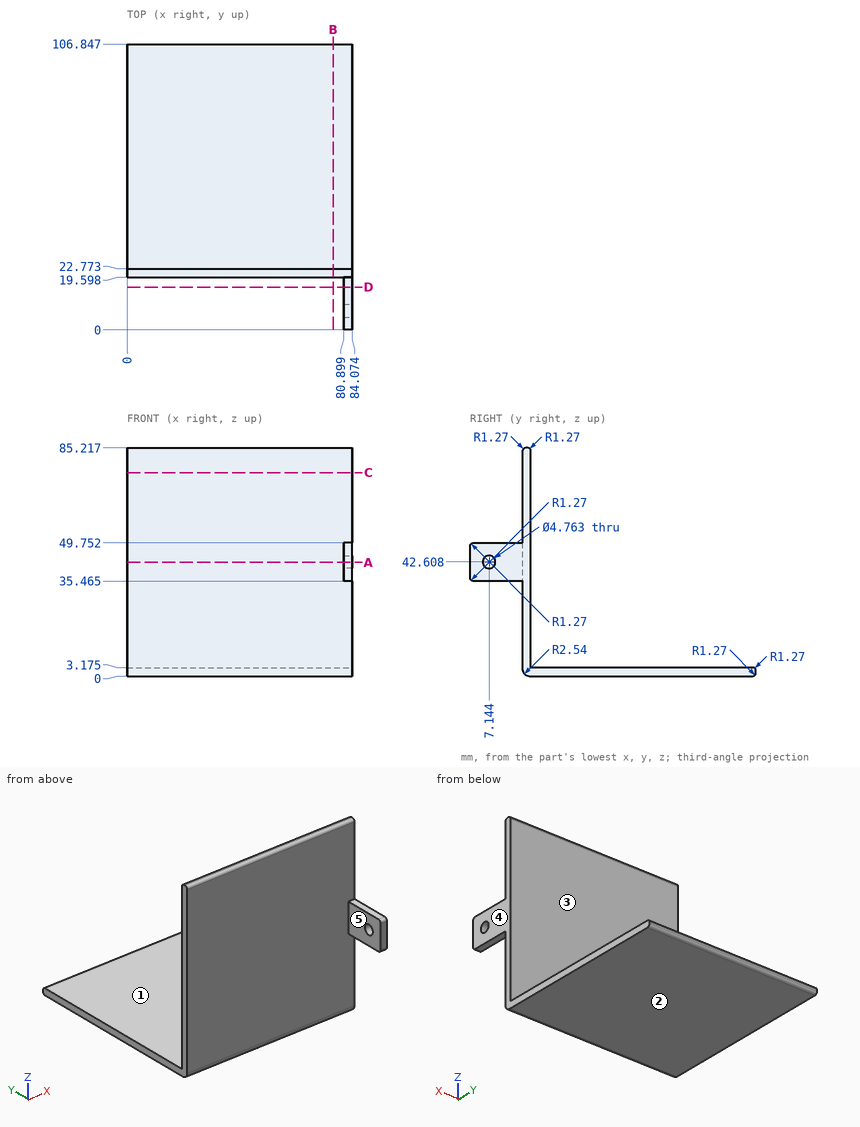
Check sheet for the drawn part. Datum: minimum x, y, z corner. Units: mm. A direction names the side the tool comes from. Give positions to 0.01 mm unless a question says otherwise; leave off trailing zeros. Order: outer loops, then holes, each group sorted by start corner. A loop starts at its lowest first (then second) coordinate and runs counter-clockwise, first axis right, second up. Notation, with made-up numbers: (44, 56.5) -> (98, 56.5) arc R11 ccw to (98, 75.5) -> close; hole circle Ø5 at (5, 86.5). An arc over 180 degrees is marked (long way). Return JSON: item names as keys, results as strings.
1. Go/stop test with flat-tipped pins: P1, Ø10, axis at y = 74.5, z = 11, coming from the -X side; P2, Ø10, axis at x = 72, z = 10.5, coming from the -Y side; P3, Ø2.5, axis at x = 82.5, y = 13, coming from the +Z side; P4, Ø11.5, axis at y = 12, z = 45, coming from the -X side. Record where each tip stops, or that it passes through.
From the geometry:
{"P1": "through", "P2": "y = 19.6", "P3": "z = 49.75", "P4": "x = 80.9"}
2. Mould release check, pull along Z, two halves, no side actions. Record for the marked faces 1, 2 and 3: +Z half, -Z half, draft (parallel to the pull), parting line (faces both ways), or undercut.
From the geometry:
{"face 1": "+Z half", "face 2": "-Z half", "face 3": "draft"}
3. Set-up check for the marked faces 4 and 5: record each of +Z, -Z, +X, -X, +Y, -Y from which the full face is reachable in a straight line by a thin tool's end or side.
From the geometry:
{"face 4": "+Z, -Z, +X, +Y, -Y", "face 5": "+Z, -Z, -X, -Y"}
4. Cross-section at A-A, the plane z = 42.5. Record the cut outline in (x, y) (1 decimal).
From the geometry:
{"outline": "(0, 19.6) -> (80.9, 19.6) -> (80.9, 9.5) -> (84.1, 9.5) -> (84.1, 22.8) -> (0, 22.8) -> close; (80.9, 0) -> (84.1, 0) -> (84.1, 4.8) -> (80.9, 4.8) -> close"}
5. Material ranges on probe 1 along Y at (x, z) = (55.5, 42.5); probe 2 along Z at (x, y) = (48.5, 47) (1 decimal); probe 3 along X at (y, z) = (12, 45.5) (1 decimal), recorded low to high. Write a range as [from, to].
From the geometry:
{"probe 1": "[19.6, 22.77]", "probe 2": "[0, 3.2]", "probe 3": "[80.9, 84.1]"}
6. Cross-section at C-C, the plane z = 76. Record the cut outline in (x, y) (1 decimal), plus the area to 3 significant figures.
From the geometry:
{"outline": "(0, 19.6) -> (84.1, 19.6) -> (84.1, 22.8) -> (0, 22.8) -> close", "area": "267 mm^2"}
7. Cross-section at B-B, the plane x = 77. Record the cut outline in (y, z) (1 decimal).
From the geometry:
{"outline": "(19.6, 2.5) arc R2.5 ccw to (22.1, 0) -> (105.6, 0) arc R1.3 ccw to (106.8, 1.3) -> (106.8, 1.9) arc R1.3 ccw to (105.6, 3.2) -> (22.8, 3.2) -> (22.8, 83.9) arc R1.3 ccw to (21.5, 85.2) -> (20.9, 85.2) arc R1.3 ccw to (19.6, 83.9) -> close"}
8. Cross-section at D-D, the plane y = 16. Record the cut outline in (x, z) (1 decimal).
From the geometry:
{"outline": "(80.9, 35.5) -> (84.1, 35.5) -> (84.1, 49.8) -> (80.9, 49.8) -> close"}
